from build123d import *

# Parameters (mm, degrees)
SKETCH1_R           = 3.25
BOSS_EXTRUDE1_DEPTH = 12.018
SKETCH6_R           = 4.8
BOSS_EXTRUDE2_DEPTH = 5
FILLET1_R           = 0.75
BOSS_EXTRUDE3_DEPTH = 1
BOSS_EXTRUDE4_DEPTH = 2


with BuildPart() as part:
    # Sketch1 → Boss-Extrude1 (new body)
    with BuildSketch(Plane(origin=(0, 0, 0), x_dir=(1, 0, 0), z_dir=(0, 1, 0))):
        with Locations(Location((0, 0, 0), (0, 0, 270))):
            Circle(SKETCH1_R)
    extrude(amount=BOSS_EXTRUDE1_DEPTH)

    # Sketch6 → Boss-Extrude2 (add)
    with BuildSketch(Plane(origin=(0, 12.018, 0), x_dir=(1, 0, 0), z_dir=(0, 1, 0))):
        with Locations(Location((0, 0, 0), (0, 0, 270))):
            Circle(SKETCH6_R)
    extrude(amount=BOSS_EXTRUDE2_DEPTH)

    # Fillet1
    fillet1_edges = [part.edges().sort_by_distance(p)[0] for p in [
        (0, 17.018, -4.8),
    ]]
    fillet(fillet1_edges, radius=FILLET1_R)

    # Sketch8 → Boss-Extrude3 (add)
    with BuildSketch(Plane(origin=(0, 17.018, 0), x_dir=(1, 0, 0), z_dir=(0, 1, 0))):
        Polygon((0, 0.75), (-3, 0.75), (-3, -0.75), (0, -0.75), (0, -1.732050808), (3, 0), (0, 1.732050808), align=None)
    extrude(amount=BOSS_EXTRUDE3_DEPTH)

    # Sketch9 → Boss-Extrude4 (add)
    with BuildSketch(Plane.XZ.offset(-12.018)):
        with BuildLine():
            Line((-4.405788806, 1.905), (-6.945788806, 1.905))
            Line((-6.945788806, 1.905), (-6.945788806, -1.905))
            Line((-6.945788806, -1.905), (-4.405788806, -1.905))
            ThreePointArc((-4.405788806, -1.905), (-4.8, 0), (-4.405788806, 1.905))
        make_face()
        with BuildLine():
            Line((4.628941564, 1.27), (7.168941564, 1.27))
            Line((7.168941564, 1.27), (7.168941564, -1.27))
            Line((7.168941564, -1.27), (4.628941564, -1.27))
            ThreePointArc((4.628941564, -1.27), (4.8, 0), (4.628941564, 1.27))
        make_face()
    extrude(amount=-BOSS_EXTRUDE4_DEPTH)


solid = part.part
CAD build for the part. Positions are in the model's coordinates, mm. A direction names the side the tool comes from. Round coordinates to 2 decimals unless told otherwise and drop trailing zeros. Loops run counter-clockwise (first coordinate to the right, second up) from the corner with the lowest first, then second, coordinate; pieces in that order, holes last. Notation, with made-up numbers: M 60,41 L 93,41 A30 cw 93,76 Z; hole C 26,9.25 d1. An arc over 180 degrees is marked long. One line per question, with ' | ' between items. Start each with the question number.
Item 1: Two-plate mould, pull along X, no slides. Class faces 1 (the cylindrical face through (-1.978, 5.925, -2.579)), 2 (the flat face through (-6, 13, -1.905)), 3 (the flat face through (-3, 17.5, 0)), 4 (the flat face through (1.479, 17.511, 0.878)): pulls with the +X half, pulls with the -X half, needs draft (parallel to the pull), parting line crosses it, or undercut.
Item 2: Which spindle directions (+Z, -Z, +X, -X, +Y, -Y) get a long thin tool onto all of the face, cutting with end or side? Do faces 5 (the flat face through (6, 13, 1.27)), 6 (the flat face through (1.521, 17.511, -0.854)), 7 (the flat face through (-1.5, 17.5, 0.75)), 8 (the flat face through (-6, 13, 1.905)), 9 (the flat face through (3.3, 12.018, -1.1)). Say none if no direction does.
Item 3: Cut at D-D, the plane y = 2.75. Write the cut outline in (x, z), plus the area to 3 significant figures.
Item 4: Cut at A-A, the plane y = 13.5. Write the cut outline in (x, z) (3 decimals).
Item 5: Pin check, flat tips, straight feed: pin 1 Ø0.5 at (y, z) = (17.5, 1.5) entering from -X; pin 2 Ø1 at (x, y) = (1, 14.5) entering from +Z; pin 3 Ø3 at (x, y) = (2.5, 14.5) entering from -Z. Stop position of each tip, or through.
Item 6: Cut at C-C, the plane x = -5.5. Write the cut outline in (y, z) (3 decimals), plus the area to 3 significant figures.
Item 7: Cut at B-B, the plane x = 5.5. Write the cut outline in (y, z).
Item 8: Wall check: line 1 (Y direction, x = -1.5, z = -1); line 2 (Y direction, x = -5.75, z = -1); line 3 (Z direction, x = -1.25, y = 12.5). Give the ranges that are in metal, low to high.
Responses:
1) face 1: parting line crosses it | face 2: needs draft | face 3: pulls with the -X half | face 4: pulls with the +X half
2) face 5: +Z, +X, +Y, -Y | face 6: -Z, +X, +Y | face 7: +Z, -X, +Y | face 8: +Z, -X, +Y, -Y | face 9: -Y
3) outline: C 0,0 d6.5 | area: 33.2 mm²
4) outline: M -6.946,-1.905 L -4.406,-1.905 A4.8 ccw 4.629,-1.27 L 7.169,-1.27 L 7.169,1.27 L 4.629,1.27 A4.8 ccw -4.406,1.905 L -6.946,1.905 Z
5) pin 1: stops at x = 0 | pin 2: stops at z = 4.77 | pin 3: stops at z = -4.69
6) outline: M 12.018,-1.905 L 14.018,-1.905 L 14.018,1.905 L 12.018,1.905 Z | area: 7.62 mm²
7) outline: M 12.02,-1.27 L 14.02,-1.27 L 14.02,1.27 L 12.02,1.27 Z
8) line 1: y = 0 to 17.02 | line 2: y = 12.02 to 14.02 | line 3: z = -4.63 to 4.63
